from build123d import *

# Parameters (mm, degrees)
SKETCH1_W               = 68.52
SKETCH1_H               = 68.52
BOSS_EXTRUDE1_DEPTH     = 35.6
SKETCH2_W               = 68.52
SKETCH2_H               = 29.4
CUT_EXTRUDE1_DEPTH      = 10.2
SKETCH3_R               = 3.2
CUT_EXTRUDE2_DEPTH      = 10.2
SKETCH4_W               = 26
SKETCH4_H               = 34.26
CUT_EXTRUDE3_DEPTH      = 25.4
CUT_EXTRUDE4_DEPTH      = 85.47542838
CUT_EXTRUDE4_DEPTH_BACK = 85.47542838
SKETCH6_R               = 2.75
SKETCH7_R               = 4.5
CUT_EXTRUDE5_DEPTH      = 13.26
CUT_EXTRUDE6_START      = -13.26
SKETCH8_R               = 4.5
CUT_EXTRUDE6_DEPTH      = 13.26


with BuildPart() as part:
    # Sketch1 → Boss-Extrude1 (new body)
    with BuildSketch(Plane.XY):
        Rectangle(SKETCH1_W, SKETCH1_H)
    extrude(amount=BOSS_EXTRUDE1_DEPTH)

    # Sketch2 → Cut-Extrude1 (cut)
    with BuildSketch(Plane.XY.offset(35.6)):
        Rectangle(SKETCH2_W, SKETCH2_H)
    extrude(amount=-CUT_EXTRUDE1_DEPTH, mode=Mode.SUBTRACT)

    # Sketch3 → Cut-Extrude2 (cut)
    with BuildSketch(Plane.XY.offset(35.6)):
        with Locations((-14, 24.2141445)):
            Circle(SKETCH3_R)
        with Locations((14, 24.2141445)):
            Circle(SKETCH3_R)
        with Locations((0, -24.2141445)):
            Circle(SKETCH3_R)
    extrude(amount=-CUT_EXTRUDE2_DEPTH, mode=Mode.SUBTRACT)

    # Sketch4 → Cut-Extrude3 (cut)
    with BuildSketch(Plane(origin=(0, 0, 0), x_dir=(-1, 0, 0), z_dir=(0, 0, -1))):
        with Locations((0, -17.13)):
            Rectangle(SKETCH4_W, SKETCH4_H)
    extrude(amount=-CUT_EXTRUDE3_DEPTH, mode=Mode.SUBTRACT)

    # Sketch6 → Cut-Extrude4 (cut, two sides: drawn at the far end of the back side and taken through both)
    with BuildSketch(Plane(origin=(34.26, 0, 0), x_dir=(0, 0, -1), z_dir=(1, 0, 0)).offset(-CUT_EXTRUDE4_DEPTH_BACK)):
        with Locations((-12.7, -7)):
            Circle(SKETCH6_R)
        with Locations((-12.7, -25)):
            Circle(SKETCH6_R)
    extrude(amount=CUT_EXTRUDE4_DEPTH + CUT_EXTRUDE4_DEPTH_BACK, mode=Mode.SUBTRACT)

    # Sketch7 → Cut-Extrude5 (cut)
    with BuildSketch(Plane(origin=(34.26, 0, 0), x_dir=(0, 0, -1), z_dir=(1, 0, 0))):
        with Locations((-12.7, -7)):
            Circle(SKETCH7_R)
        with Locations((-12.7, -25)):
            Circle(SKETCH7_R)
    extrude(amount=-CUT_EXTRUDE5_DEPTH, mode=Mode.SUBTRACT)

    # Sketch8 → Cut-Extrude6 (cut)
    with BuildSketch(Plane.ZY.offset(34.26).offset(CUT_EXTRUDE6_START)):
        with Locations(Location((12.7, -7, 0), (0, 0, 180))):
            Circle(SKETCH8_R)
        with Locations(Location((12.7, -25, 0), (0, 0, 180))):
            Circle(SKETCH8_R)
    extrude(amount=CUT_EXTRUDE6_DEPTH, mode=Mode.SUBTRACT)


solid = part.part
CAD build for the part. Positions are in the model's coordinates, mm. A direction names the side the tool comes from. Coordinates: 2 decimals unless noted, no trailing zeros. Write each loop counter-clockwise with the first axis right and the second up, starting at its lowest first coordinate (ties: lowest second). Pieces come first, ordered by that corner, then holes. Notation, with made-up numbers: M 64.5,-27 L 74.5,-27 A35 ccw 74.5,10 Z; hole C 77,42.25 d7. An arc over 180 degrees is marked long. Answer as a JSON object with one key per item and string values. Group by question number.
1) Saw through at B-B (y = -13.5). Write the cut outline in (x, z), plus the area to 3 significant figures.
2) Pin check, flat tips, straight feed: pin 1 Ø5 at (y, z) = (0, 30) entering from +X; pin 2 Ø2.5 at (y, z) = (-7, 14.5) entering from -X; pin 3 Ø4 at (x, y) = (4, -23.5) entering from -Z; pin 4 Ø5 at (x, y) = (-26, -0.5) entering from +Z. Stop position of each tip, or through.
3) Tool access for faces 4 (the face through (3, -22, 25.4)), 5 (the face through (14, 24, 25.4)), 6 (the face through (-0.5, 0.2, 25.4)): list every direction of +Z, -Z, +X, -X, +Y, -Y with a clear straight run to the whole face (end or side of a thin tool).
4) Saw through at A-A (x = 0). Write the cut outline in (y, z), plus the area to 3 significant figures.
5) Mould opens along Y. For faces 1 (the face through (-13, -17, 13)), 2 (the face through (0, 0, 13)), 3 (the face through (-27.537, -28.794, 10.281)) say: +Y half, -Y half, draft (parallel to the pull), parting line (faces both ways), or undercut.
6) Saw through at C-C (x = -7). Write the cut outline in (y, z), plus the area to 3 significant figures.
7) Wall check: line 1 (Y direction, x = -18.5, z = 12.7); line 2 (Y direction, x = -24.75, z = 12.7); line 3 (Z direction, x = -25.75, y = -25). Give the ranges that are in metal, low to high. Write a range as from..to.
8) Saw through at D-D (x = 14). Write the cut outline in (y, z), plus the area to 3 significant figures.
Values follow:
{
 "1": {"outline": "M -34.26,0 L -13,0 L -13,25.4 L -34.26,25.4 Z; M 13,0 L 34.26,0 L 34.26,25.4 L 13,25.4 Z", "area": "1,080 mm2"},
 "2": {"pin 1": "passes through", "pin 2": "stops at x = -21", "pin 3": "stops at z = 25.4", "pin 4": "stops at z = 25.4"},
 "3": {"face 4": "-Z, -Y", "face 5": "+Z", "face 6": "+Z, +X, -X"},
 "4": {"outline": "M -34.26,25.4 L -27.41,25.4 L -27.41,35.6 L -34.26,35.6 Z; M -21.01,25.4 L -14.7,25.4 L -14.7,35.6 L -21.01,35.6 Z; M 0,0 L 34.26,0 L 34.26,35.6 L 14.7,35.6 L 14.7,25.4 L 0,25.4 Z", "area": "1,200 mm2"},
 "5": {"face 1": "draft", "face 2": "-Y half", "face 3": "undercut"},
 "6": {"outline": "M -34.26,25.4 L -14.7,25.4 L -14.7,35.6 L -34.26,35.6 Z; M 0,0 L 34.26,0 L 34.26,35.6 L 14.7,35.6 L 14.7,25.4 L 0,25.4 Z", "area": "1,270 mm2"},
 "7": {"line 1": "y = -34.26..-27.75, -22.25..-9.75, -4.25..34.26", "line 2": "y = -34.26..-29.5, -20.5..-11.5, -2.5..34.26", "line 3": "z = 0..8.2, 17.2..35.6"},
 "8": {"outline": "M -34.26,0 L 34.26,0 L 34.26,35.6 L 27.41,35.6 L 27.41,25.4 L 21.01,25.4 L 21.01,35.6 L 14.7,35.6 L 14.7,25.4 L -14.7,25.4 L -14.7,35.6 L -34.26,35.6 Z; hole C -25,12.7 d5.5; hole C -7,12.7 d5.5", "area": "2,030 mm2"}
}
